```python
from build123d import *

# Parameters (mm, degrees)
SKETCH_1_W          = 10
SKETCH_1_H          = 10
SKETCH_1_W_2        = 8
SKETCH_1_H_2        = 8
EXTRUDE_1_DEPTH     = 499
SKETCH_2_R          = 2
CUT_EXTRUDE_1_DEPTH = 500.125234786
SKETCH_3_R          = 2.1
CUT_EXTRUDE_2_DEPTH = 500.125234786


with BuildPart() as part:
    # ｽｹｯﾁ1 → 押し出し-薄板1 (new body)
    with BuildSketch(Plane.XY):
        Rectangle(SKETCH_1_W, SKETCH_1_H)
        Rectangle(SKETCH_1_W_2, SKETCH_1_H_2, mode=Mode.SUBTRACT)
    extrude(amount=EXTRUDE_1_DEPTH)

    # ｽｹｯﾁ2 → ｶｯﾄ - 押し出し1 (cut, through all)
    with BuildSketch(Plane(origin=(0, 5, 0), x_dir=(1, 0, 0), z_dir=(0, 1, 0))):
        with Locations(Location((0, -5, 0), (0, 0, 270))):
            Circle(SKETCH_2_R)
        with Locations(Location((0, -394.5, 0), (0, 0, 270))):
            Circle(SKETCH_2_R)
    extrude(amount=-CUT_EXTRUDE_1_DEPTH, mode=Mode.SUBTRACT)

    # ｽｹｯﾁ3 → ｶｯﾄ - 押し出し2 (cut, through all)
    with BuildSketch(Plane(origin=(5, 0, 0), x_dir=(0, 0, -1), z_dir=(1, 0, 0))):
        with Locations((-485.96, 0)):
            Circle(SKETCH_3_R)
    extrude(amount=-CUT_EXTRUDE_2_DEPTH, mode=Mode.SUBTRACT)


solid = part.part
```
Here's how the part is built. I have some questions about the finished solid (model axes, mm). A direction names the side the tool comes from. Coordinates: 2 decimals unless noted, no trailing zeros. Write each loop counter-clockwise with the first axis right and the second up, starting at its lowest first coordinate (ties: lowest second). Pieces come first, ordered by that corner, then holes. Notation, with made-up numbers: (78, 33.25) - (102, 33.25) arc R24 cw to (102, 54.25) - close; hole circle Ø10 at (-14.75, -18.75). An arc over 180 degrees is marked (long way). One line per item, written item: value.
1) We'd pull the mould along Y, two halves only. Please class faces 3 (the flat face through (0, -5, 246)), 4 (the flat face through (4, 0, 246)), 5 (the flat face through (5, 0, 246)): pulls with the +Y half, pulls with the -Y half, needs draft (parallel to the pull), parting line crosses it, or undercut.
Model answer:
face 3: pulls with the -Y half
face 4: undercut
face 5: needs draft
2) I need wall thicknesses on line 1 along Y through (x, z) = (-3.75, 76.5); line 2 along X through (y, z) = (4.65, 394.5). Which ranges of each line are inside material? Lowest first, please.
Model answer:
line 1: y = -5 to -4, 4 to 5
line 2: x = -5 to -2, 2 to 5
3) On a 3-axis mill with a long thin cutter (end or side, diameter ignored), from which of +Z, -Z, +X, -X, +Y, -Y can I reach the whole of each face in a straight line? I mean faces 1 (the flat face through (-4.5, 0.1, 0)), 2 (the flat face through (0, 4, 246)). Say none if no direction works.
Model answer:
face 1: -Z, +X, -X, +Y, -Y
face 2: +Z, -Z
4) Suppose I cut it at A-A on y = 0. Write out the boundary of the cut face in (x, z), and give its area (3 significant figures).
Model answer:
outline: (-5, 0) - (-4, 0) - (-4, 483.86) - (-5, 483.86) - close; (-5, 488.06) - (-4, 488.06) - (-4, 499) - (-5, 499) - close; (4, 0) - (5, 0) - (5, 483.86) - (4, 483.86) - close; (4, 488.06) - (5, 488.06) - (5, 499) - (4, 499) - close
area: 990 mm²
5) Suppose I cut it at B-B on z = 116. Write out the boundary of the cut face in (x, y), and give its area (3 significant figures).
Model answer:
outline: (-5, -5) - (5, -5) - (5, 5) - (-5, 5) - close; hole (-4, -4) - (4, -4) - (4, 4) - (-4, 4) - close
area: 36.0 mm²
6) I'm going to push a flat-ended pin straight in: P1, Ø5, axis at x = 0, z = 394.5, coming from the +Y side. Where does the tip first touch, or does it pass through?
Model answer:
P1: stops at y = 5
